```python
from build123d import *

# Parameters (mm, degrees)
F0_R     = 5
F1_DEPTH = 2.5
F2_DEPTH = 10
F3_DEPTH = 10


with BuildPart() as f1:
    # F0 (on Top) → F1 (new body, symmetric)
    with BuildSketch(Plane.XY):
        with BuildLine():
            Line((-15, -10), (15, -10))
            ThreePointArc((15, -10), (25, 0), (15, 10))
            Line((15, 10), (-15, 10))
            ThreePointArc((-15, 10), (-25, 0), (-15, -10))
        make_face()
        with Locations((-15, 0)):
            Circle(F0_R, mode=Mode.SUBTRACT)
        with Locations((15, 0)):
            Circle(F0_R, mode=Mode.SUBTRACT)
        with Locations((-15, 0)):
            Circle(F0_R)
        with Locations((15, 0)):
            Circle(F0_R)
    extrude(amount=F1_DEPTH, both=True)

    # F0 (on Top) → F2 (join)
    with BuildSketch(Plane.XY):
        with Locations((-15, 0)):
            Circle(F0_R)
    extrude(amount=F2_DEPTH)

    # F0 (on Top) → F3 (join)
    with BuildSketch(Plane.XY):
        with Locations((15, 0)):
            Circle(F0_R)
    extrude(amount=-F3_DEPTH)


solid = f1.part
```
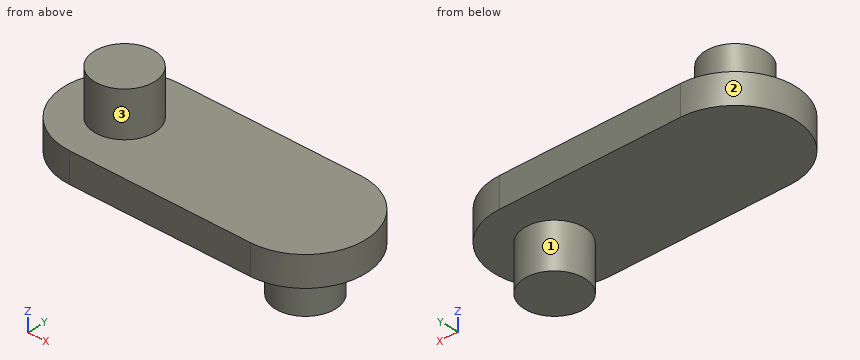
Source: CAD feature listing. Evaluate the final solid. Frame: model axes, mm. Face numbers are marked on the shaded views. A direction names the side the tool comes from. Round coordinates to 2 decimals unless told otherwise and drop trailing zeros. Loops run counter-clockwise (first coordinate to the right, second up) from the corner with the lowest first, then second, coordinate; pieces in that order, holes last. Notation, with made-up numbers: M 76.25,78 L 128.25,78 A21 ccw 128.25,97 Z; hole C -2.5,61 d1. An arc over 180 degrees is marked long. Use a Markdown table: item, result. Add a question column.
1. Cut plane B-B, the plane z = 8. Output: boundary loops of the cut face in (x, y), and give its area (3 significant figures).
2. Cut plane C-C, the plane x = 11.5. Output: boundary loops of the cut face in (y, z), and give its area (3 significant figures).
3. Cut plane A-A, the plane y = 0. Output: boundary loops of the cut face in (x, z), and give its area (3 significant figures).
4. Ray query, line 1 along Z through (x, y) = (18, 3.75); line 2 along Z through (x, y) = (-3.5, -7.5); line 3 along X through (y, z) = (-6, -2). Return the intervals inside material, ascending. Write a range as [from, to].
5. Contact query for flat-ended pins moving along their axis: pin 1 (4 mm diameter, centred on y = -7.5, z = 5, fed in from -X); pin 2 (10 mm diameter, centred on x = 0, y = -1, fed in from -Z); pin 3 (4 mm diameter, centred on y = 5.5, z = -7, fed in from -X); pin 4 (6 mm diameter, centred on y = 6, z = 0, fed in from -X). Output: stop coordinate, or through.
6. Cut plane D-D, the plane y = 3. Output: boundary loops of the cut face in (x, z), and give its area (3 significant figures).
7. Set-up query: the marked faces 1, 2 and 3. Return all of +Z, -Z, +X, -X, +Y, -Y with unobstructed straight access to the full face (end or side cutting, diameter ignored); none if empty.
Solution:
| question | item | result |
|---|---|---|
| 1 | outline | C -15,0 d10 |
| 1 | area | 78.5 mm2 |
| 2 | outline | M -10,-2.5 L -3.57,-2.5 L -3.57,-10 L 3.57,-10 L 3.57,-2.5 L 10,-2.5 L 10,2.5 L -10,2.5 Z |
| 2 | area | 154 mm2 |
| 3 | outline | M -25,-2.5 L 10,-2.5 L 10,-10 L 20,-10 L 20,-2.5 L 25,-2.5 L 25,2.5 L -10,2.5 L -10,10 L -20,10 L -20,2.5 L -25,2.5 Z |
| 3 | area | 400 mm2 |
| 4 | line 1 | z = [-10, 2.5] |
| 4 | line 2 | z = [-2.5, 2.5] |
| 4 | line 3 | x = [-23, 23] |
| 5 | pin 1 | passes through |
| 5 | pin 2 | stops at z = -2.5 |
| 5 | pin 3 | stops at x = 11.43 |
| 5 | pin 4 | stops at x = -24.54 |
| 6 | outline | M -24.54,-2.5 L 11,-2.5 L 11,-10 L 19,-10 L 19,-2.5 L 24.54,-2.5 L 24.54,2.5 L -11,2.5 L -11,10 L -19,10 L -19,2.5 L -24.54,2.5 Z |
| 6 | area | 365 mm2 |
| 7 | face 1 | -Z |
| 7 | face 2 | +Z, -Z, -X |
| 7 | face 3 | +Z |
